Part print with two shaded views. Sizes in mm from the minimum x, y, z corner. Round coordinates to 2 decimals unless told otherwise and drop trailing zeros. Write each loop counter-clockwise with the first axis right and the second up, starting at its lowest first coordinate (ties: lowest second). Pieces come first, ordered by that corner, then holes. Notation, with made-up numbers: (-10, 43.5) - (31, 43.5) arc R30 ccw to (31, 74.5) - close; hole circle Ø3 at (34, 31.25). An arc over 180 degrees is marked (long way). Answer as a JSON object with one key per item and string values. Group by question number.
Item 1: Slice it at D-D, the plane x = 11.5. List the corners of the cut face in (y, z).
Item 2: Two-plate mould, pull along Z, no slides. Class the marked faces 1, 2 and 3: +Z half, -Z half, draft (parallel to the pull), parting line (faces both ways), or undercut.
Item 3: Probe line 1 (Z direction, x = 54.5, y = 29) (1 decimal); line 2 (X direction, y = 13, z = 17.5) (1 decimal); line 3 (Z direction, x = 20.5, y = 4) (1 decimal). List the from-to ranges inside material, lowest first. Write a range as from..to.
Item 4: Flat gauge pin, fed straight in: pin 1 (8 mm diameter, centred on y = 26.5, z = 47.5, fed in from -X). Where does the tip first touch, or does it go through?
Item 5: Slice it at A-A, the plane x = 54.5. Give the number of separate pieces and of enclosed holes in the cut face, then the cut area to 3 significant figures.
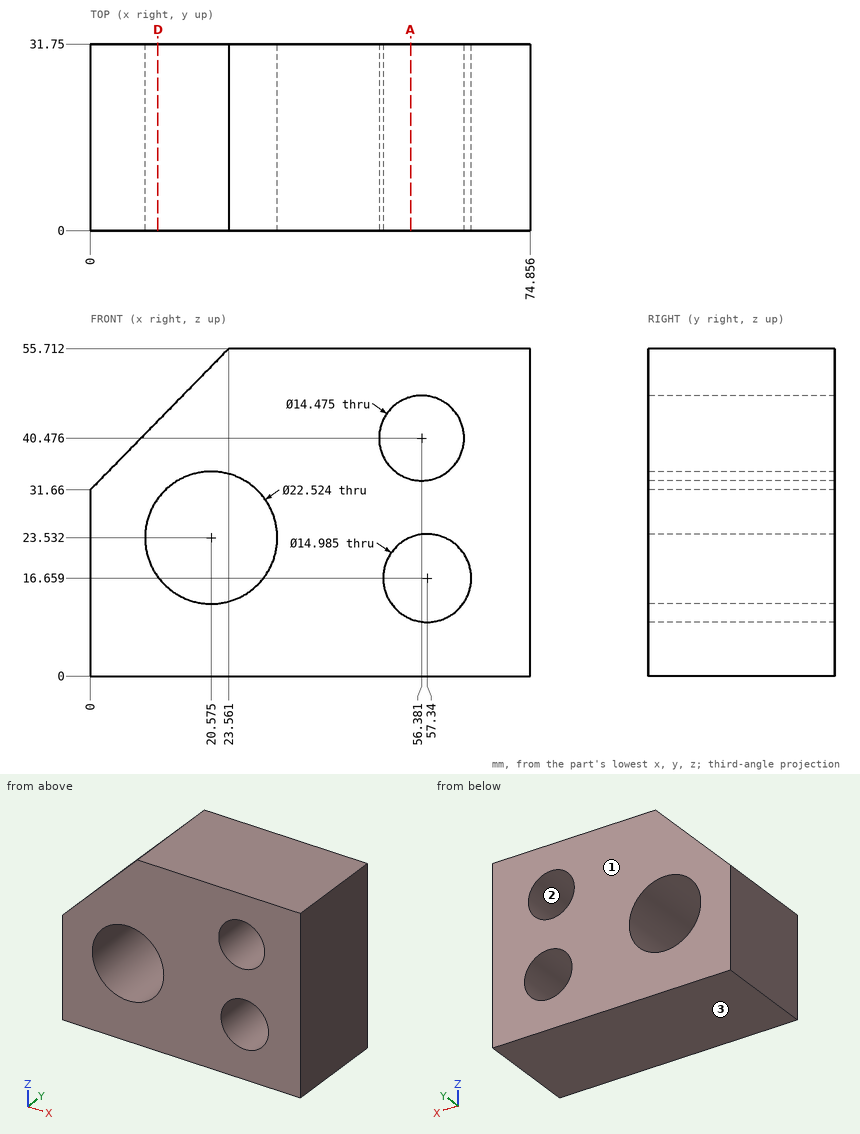
Geometry says:
{
 "1": {"outline": "(0, 0) - (31.75, 0) - (31.75, 16.86) - (0, 16.86) - close; (0, 30.2) - (31.75, 30.2) - (31.75, 43.4) - (0, 43.4) - close"},
 "2": {"face 1": "draft", "face 2": "undercut", "face 3": "-Z half"},
 "3": {"line 1": "z = 0..9.7, 23.6..33.5, 47.5..55.7", "line 2": "x = 0..11.1, 30.1..49.9, 64.8..74.9", "line 3": "z = 0..12.3, 34.8..52.6"},
 "4": {"pin 1": "stops at x = 11.6"},
 "5": {"separate pieces": "3", "enclosed holes": "0", "area": "885 mm^2"}
}
